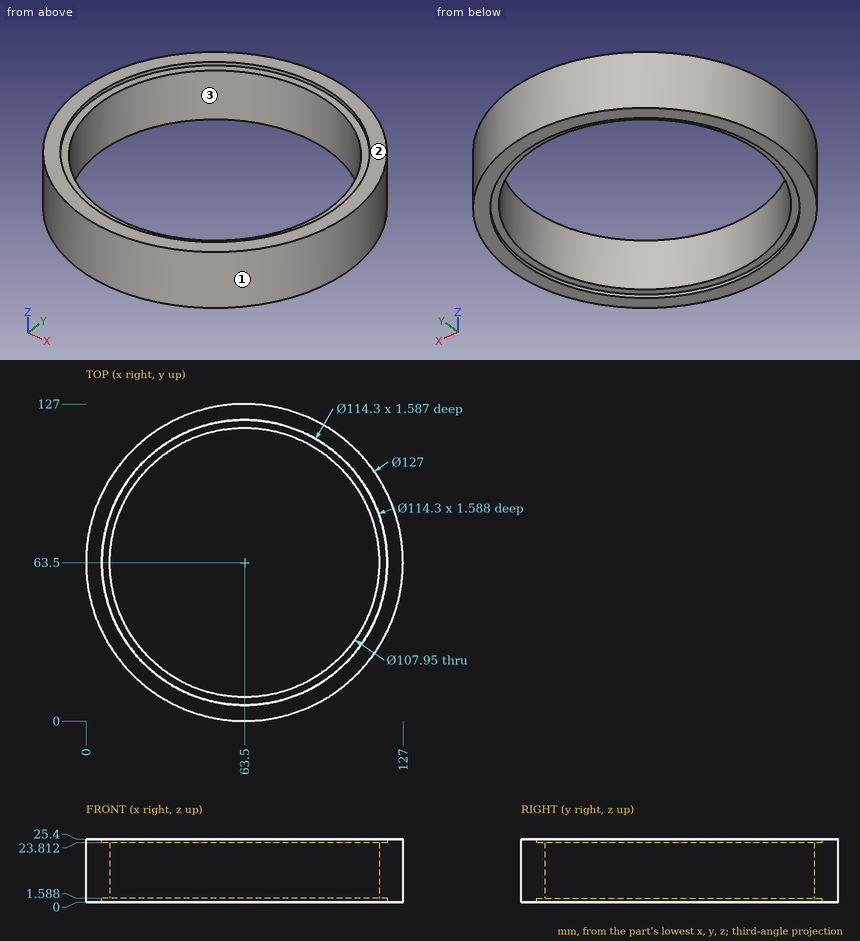
Geometry check sheet. Reference: drawing and pictorial views, mm from the part's lowest x, y, z. Give positions to 0.01 mm unless a question says otherwise; leave off trailing zeros. Use CSV: the item, a comma, the result in double quotes. Start each with the question number.
1) Material ranges on line 1 (Y direction, x = 63.5, z = 0.5); line 2 (Y direction, x = 63.5, z = 9.25) (1 decimal); line 3 (X direction, y = 64, z = 22.5), recorded low to high. Write a range as from..to.
2) Go/stop test with flat-tipped pins: P1, Ø1, axis at y = 72, z = 17.5, coming from the +X side; P2, Ø12, axis at x = 80, z = 19, coming from the -Y side; P3, Ø1, axis at x = 45, z = 10, coming from the -Y side (1 decimal). Record where each tip stops, or that it passes through.
3) Mould release check, pull along Y, two halves, no side actions. Record for the marked faces 1, 2 and 3: released by +Y, released by -Y, zero draft, split by the parting line, or undercut.
Recorded:
1,line 1,"0..6.35, 120.65..127"
1,line 2,"0..9.5, 117.5..127"
1,line 3,"0..9.53, 117.47..127"
2,P1,"x = 126.49"
2,P2,"y = 0.87"
2,P3,"y = 2.6"
3,face 1,"split by the parting line"
3,face 2,"zero draft"
3,face 3,"undercut"
